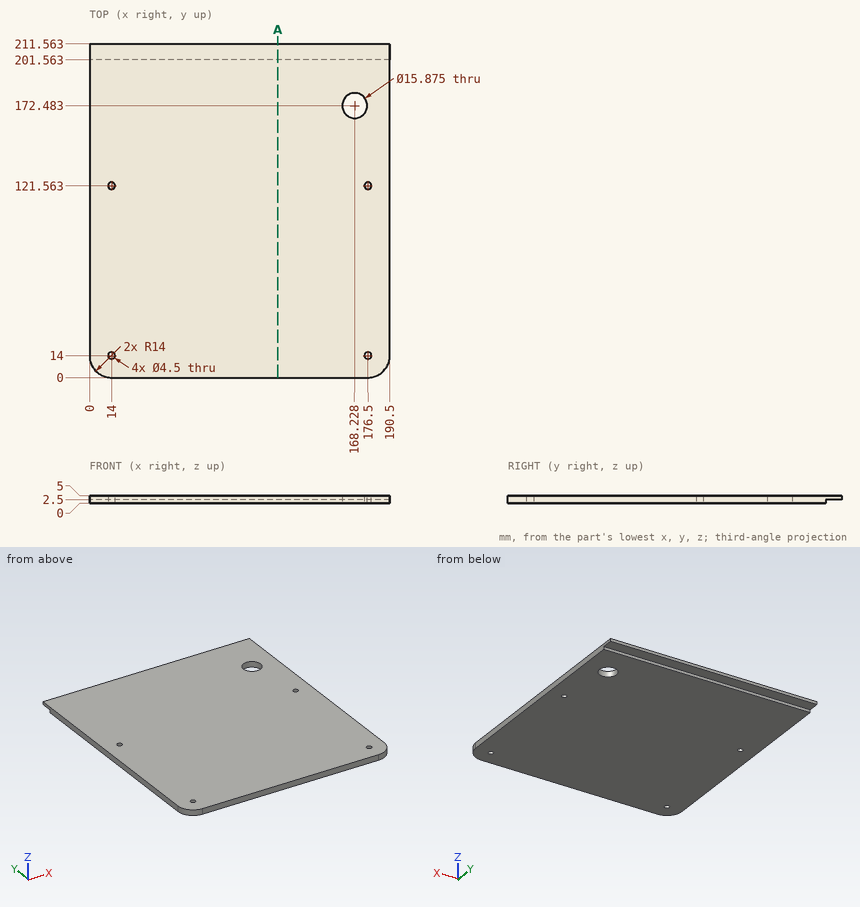
Geometry: see drawing. Coordinates: mm, zero at the bounding-box minimum. Give positions to 0.01 mm unless a question says otherwise; leave off trailing zeros. Write each loop counter-clockwise with the first axis right and the second up, starting at its lowest first coordinate (ties: lowest second). Pieces come first, ordered by that corner, then holes. Notation, with made-up numbers: M -14.5,23.25 L 7.5,23.25 A23 ccw 7.5,39.25 Z; hole C 41,39.25 d1. An arc over 180 degrees is marked long. Answer in a Markdown table with one row per item. Add a question column.
(1) Ray query, line 1 (Y direction, x = 14, z = 1.6); line 2 (X direction, y = 121.5, z = 0.9); line 3 (Y direction, x = 176.5, z = 2.95). Return the intervals inside material, ascending.
(2) First-contact query: pin 1 (3.5 mm diameter, centred on x = 176.5, y = 14, fed in from -Z); pin 2 (0.8 mm diameter, centred on x = 92.5, z = 1, fed in from +Y); pin 3 (8 mm diameter, centred on x = 93.5, y = 207, fed in from -Z). Flat tips, straight axial feed; report the tip coordinate or a pass-through.
(3) Section A-A on x = 119.5. Return loops of the section in (y, z), and give its area (3 significant figures).
Result set:
| question | item | result |
|---|---|---|
| 1 | line 1 | y = 0 to 11.75, 16.25 to 119.31, 123.81 to 201.56 |
| 1 | line 2 | x = 0 to 11.75, 16.25 to 174.25, 178.75 to 190.5 |
| 1 | line 3 | y = 0 to 11.75, 16.25 to 119.31, 123.81 to 211.56 |
| 2 | pin 1 | passes through |
| 2 | pin 2 | stops at y = 201.56 |
| 2 | pin 3 | stops at z = 2.5 |
| 3 | outline | M 0,0 L 201.56,0 L 201.56,2.5 L 211.56,2.5 L 211.56,5 L 0,5 Z |
| 3 | area | 1,030 mm^2 |
